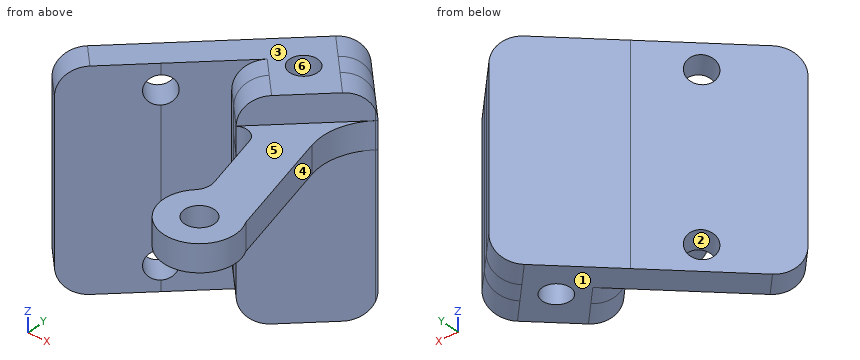
from build123d import *

# Parameters (mm, degrees)
SKETCH_1_R           = 1.55
SKETCH_1_R_2         = 1.65
EXTRUDE_1_DEPTH      = 3
EXTRUDE_5_DEPTH      = 3
EXTRUDE_5_DEPTH_BACK = 20.5
SKETCH_2_R           = 1.55
SKETCH_3_W           = 2.999466183
SKETCH_3_H           = 23.5
EXTRUDE_9_DEPTH      = 15
CUT_EXTRUDE_1_DEPTH  = 43.137686458
CUT_EXTRUDE_2_DEPTH  = 41.555271529
SKETCH_6_R           = 1.55
CUT_EXTRUDE_3_DEPTH  = 10
FILLET_1_R           = 3
FILLET_2_R           = 3
FILLET_3_R           = 3


with BuildPart() as part:
    # 草图1 → 凸台-拉伸1 (new body)
    with BuildSketch(Plane(origin=(0, 0, -3.362857667), x_dir=(-1, 0, 0), z_dir=(0, 0, -1))):
        with BuildLine():
            Line((-8.929456987, 17.45330102), (-12.208534908, 5.216337034))
            ThreePointArc((-12.208534908, 5.216337034), (-8.203956956, -0.691485495), (-5.819308033, 6.03550946))
            ThreePointArc((-5.819308033, 6.03550946), (-6.310108859, 6.921233679), (-6.304159928, 7.933833034))
            Line((-6.304159928, 7.933833034), (-4.539684391, 14.518557193))
            ThreePointArc((-4.539684391, 14.518557193), (-3.62301138, 15.532716808), (-2.264294404, 15.382060533))
            Line((-2.264294404, 15.382060533), (-0.142530428, 17.503217343))
            Line((-0.142530428, 17.503217343), (4.099819599, 13.25965297))
            Line((4.099819599, 13.25965297), (5.797509256, 14.956856814))
            Line((5.797509256, 14.956856814), (1.554532399, 19.201048196))
            Line((1.554532399, 19.201048196), (3.675778765, 21.321687543))
            Line((3.675778765, 21.321687543), (-4.808443123, 29.808337985))
            Line((-4.808443123, 29.808337985), (-6.931968366, 27.685420414))
            Line((-6.931968366, 27.685420414), (-11.173246227, 31.927912314))
            Line((-11.173246227, 31.927912314), (-12.870428791, 30.231215419))
            Line((-12.870428791, 30.231215419), (-8.629080401, 25.98865297))
            Line((-8.629080401, 25.98865297), (-10.749072595, 23.869267436))
            Line((-10.749072595, 23.869267436), (-10.611098311, 23.731253658))
            ThreePointArc((-10.611098311, 23.731253658), (-8.929299443, 20.817545637), (-8.929456987, 17.45330102))
        make_face()
        with Locations(Location((-3.536567574, 22.593983824, 0), (0, 0, 180))):
            Circle(SKETCH_1_R, mode=Mode.SUBTRACT)
        with Locations(Location((-8.71249984, 3.274951558, 0), (0, 0, 180))):
            Circle(SKETCH_1_R_2, mode=Mode.SUBTRACT)
    extrude(amount=-EXTRUDE_1_DEPTH)

    # 草图2 → 凸台-拉伸5 (add, two sides: drawn at the far end of the back side and taken through both)
    with BuildSketch(Plane.XY.offset(-0.362857667).offset(-EXTRUDE_5_DEPTH_BACK)):
        Polygon((6.931968366, 27.685420414), (4.808443123, 29.808337985), (-3.675778765, 21.321687543), (-1.554532399, 19.201048196), (-1.554756221, 19.20082431), (-5.797509256, 14.956856814), (-4.099819599, 13.25965297), (0.142530428, 17.503217343), (0.142754305, 17.503441284), (2.264294404, 15.382060533), (10.611098311, 23.731253658), (10.748516293, 23.868710975), (10.749072595, 23.869267436), (8.629080401, 25.98865297), (12.870358263, 30.23114487), (11.173246227, 31.927912314), align=None)
        with Locations((3.536567574, 22.593983824)):
            Circle(SKETCH_2_R, mode=Mode.SUBTRACT)
    extrude(amount=EXTRUDE_5_DEPTH + EXTRUDE_5_DEPTH_BACK)

    # 草图3 → 凸台-拉伸9 (add)
    with BuildSketch(Plane(origin=(8.823479961, 8.826005625, 0), x_dir=(0.7072079618145243, -0.7070055860784599, 0), z_dir=(-0.7070055860784599, -0.7072079618145243, 0))):
        with Locations((-16.174359114, -9.112857667)):
            Rectangle(SKETCH_3_W, SKETCH_3_H)
    extrude(amount=EXTRUDE_9_DEPTH)

    # 草图4 → 切除-拉伸1 (cut, through all)
    with BuildSketch(Plane(origin=(0, 0, -20.862857667), x_dir=(-1, 0, 0), z_dir=(0, 0, -1))):
        Polygon((-11.306274604, 32.060978769), (-13.003386639, 30.364211325), (-8.629080401, 25.98865297), (-6.931968366, 27.685420414), align=None)
    extrude(amount=-CUT_EXTRUDE_1_DEPTH, mode=Mode.SUBTRACT)

    # 草图5 → 切除-拉伸2 (cut, through all)
    with BuildSketch(Plane(origin=(0, 0, -20.862857667), x_dir=(-1, 0, 0), z_dir=(0, 0, -1))):
        Polygon((-0.142754305, 17.503441284), (4.099819599, 13.25965297), (5.797509256, 14.956856814), (1.554935352, 19.200645127), align=None)
    extrude(amount=-CUT_EXTRUDE_2_DEPTH, mode=Mode.SUBTRACT)

    # 草图6 → 切除-拉伸3 (cut)
    with BuildSketch(Plane(origin=(-10.37801236, 10.375042572, 0), x_dir=(0, 0, -1), z_dir=(0.7072079618145242, -0.7070055860784599, 0))):
        with Locations(Location((0.112857667, 6.48007107, 0), (0, 0, 90))):
            Circle(SKETCH_6_R)
        with Locations(Location((18.112857667, 6.48007107, 0), (0, 0, 90))):
            Circle(SKETCH_6_R)
    extrude(amount=-CUT_EXTRUDE_3_DEPTH, mode=Mode.SUBTRACT)

    # 圆角1
    fillet_1_edges = [part.edges().sort_by_distance(p)[0] for p in [
        (-0.706090524, 18.352043206, 2.637142333),
        (-0.706090524, 18.352043206, -20.862857667),
        (1.203524355, 16.442750908, -20.862857667),
        (1.203524355, 16.442750908, 2.637142333),
    ]]
    fillet(fillet_1_edges, radius=FILLET_1_R - 0.0001)  # a hair under: the kernel refuses the full size

    # 圆角2
    fillet_2_edges = [part.edges().sort_by_distance(p)[0] for p in [
        (7.780524383, 26.837036692, 2.637142333),
        (7.780524383, 26.837036692, -20.862857667),
        (9.689076498, 24.928960203, -20.862857667),
        (5.870205744, 28.746879199, -20.862857667),
        (9.689076498, 24.928960203, 2.637142333),
        (5.870205744, 28.746879199, 2.637142333),
    ]]
    fillet(fillet_2_edges, radius=FILLET_2_R)

    # 圆角3
    fillet_3_edges = [part.edges().sort_by_distance(p)[0] for p in [
        (-13.220239373, 9.653248443, -20.862857667),
        (-13.220239373, 9.653248443, 2.637142333),
    ]]
    fillet(fillet_3_edges, radius=FILLET_3_R)


solid = part.part
Geometry: final body of the model. Coordinates: model frame, mm. Face numbers are marked on the shaded views. A direction names the side the tool comes from. Give positions to 0.01 mm unless a question says otherwise; leave off trailing zeros. Write each loop counter-clockwise with the first axis right and the second up, starting at its lowest first coordinate (ties: lowest second). Pieces come first, ordered by that corner, then holes. Notation, with made-up numbers: (7.25, -7) - (29.25, -7) arc R10 cw to (29.25, 4) - close; hole circle Ø3 at (71.5, 38.5). An arc over 180 degrees is marked (long way). Return JSON: item names as keys, results as strings. Group by question number.
1) Mould query, pull axis Z, two halves, no side actions, for the marked faces 1, 2 and 3. Classes: released by +Z, released by -Z, zero draft, split by the parting line, or undercut.
2) Line query: line 1 (X direction, y = 18, z = -7.75); line 2 (Y direction, x = 4.25, z = -5.5); line 3 (X direction, y = 22.5, z = -8). Output: solid intervals per line, ascending.
3) First-contact query: P1, Ø1, axis at x = 8, y = 23.5, coming from the +Z side; P2, Ø5, axis at x = 5.5, y = 8, coming from the -Z side; P3, Ø12, axis at y = 24.5, z = -9.5, coming from the -X side; P4, Ø3, axis at x = 8.71, y = 3.27, coming from the -Z side. Flat tips, straight axial feed; report the tip coordinate or a pass-through.
4) Section D-D on x = -2. Return the cut outline in (y, z), plus the area to 3 significant figures.
5) Section B-B on y = 4. Return the cut outline in (x, z).
6) Section C-C on z = -2.25. State how many separate pieces and enclosed holes the cut face has, plus the area to 3 significant figures.
7) Set-up query: the marked faces 4, 5 and 6. Return all of +Z, -Z, +X, -X, +Y, -Y with unobstructed straight access to the full face (end or side cutting, diameter ignored); none if empty.
Filled in:
{
 "1": {"face 1": "released by -Z", "face 2": "undercut", "face 3": "released by +Z"},
 "2": {"line 1": "x = -7 to -2.76, -0.35 to 4.88", "line 2": "y = 17.37 to 21.22, 23.97 to 29.25", "line 3": "x = -2.5 to 1.99, 5.08 to 9.38"},
 "3": {"P1": "stops at z = 2.62", "P2": "stops at z = -3.36", "P3": "stops at x = -6.5", "P4": "passes through"},
 "4": {"outline": "(18.76, -20.86) - (23, -20.86) - (23, 2.64) - (18.76, 2.64) - close", "area": "99.7 mm^2"},
 "5": {"outline": "(4.78, -3.36) - (7.23, -3.36) - (7.23, -0.36) - (4.78, -0.36) - close; (10.19, -3.36) - (12.65, -3.36) - (12.65, -0.36) - (10.19, -0.36) - close"},
 "6": {"separate pieces": "1", "enclosed holes": "2", "area": "247 mm^2"},
 "7": {"face 4": "+Z, -Z, +X", "face 5": "+Z, +X, -Y", "face 6": "+Z, -Z"}
}
